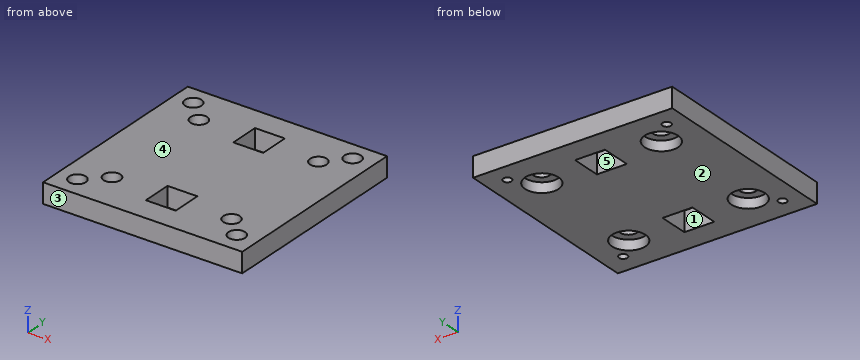
```python
from build123d import *

# Parameters (mm, degrees)
SKETCH044_W     = 100
SKETCH044_H     = 100
PAD009_DEPTH    = 10
SKETCH047_R     = 2.1
POCKET036_DEPTH = 10
SKETCH048_R     = 4.2
POCKET037_DEPTH = 5
SKETCH045_R     = 4.2
SKETCH045_W     = 15
SKETCH045_H     = 15
POCKET038_DEPTH = 10
SKETCH046_R     = 8.4
POCKET039_DEPTH = 5


with BuildPart() as part:
    # Sketch044 → Pad009 (new body)
    with BuildSketch(Plane.XY):
        with Locations((278.148773, 55.911007)):
            Rectangle(SKETCH044_W, SKETCH044_H)
    extrude(amount=PAD009_DEPTH)

    # Sketch047 → Pocket036 (cut)
    with BuildSketch(Plane.XY.offset(10)):
        with Locations((237.948565, 96.209783)):
            Circle(SKETCH047_R)
        with Locations((317.948565, 96.209783)):
            Circle(SKETCH047_R)
        with Locations((237.948565, 16.209783)):
            Circle(SKETCH047_R)
        with Locations((317.948565, 16.209783)):
            Circle(SKETCH047_R)
    extrude(amount=-POCKET036_DEPTH, mode=Mode.SUBTRACT)

    # Sketch048 (on Face5 of Pocket036) → Pocket037 (cut)
    with BuildSketch(Plane.XY.offset(10)):
        with Locations((237.975067, 96.170716)):
            Circle(SKETCH048_R)
        with Locations((317.975067, 96.170716)):
            Circle(SKETCH048_R)
        with Locations((237.975067, 16.170716)):
            Circle(SKETCH048_R)
        with Locations((317.975067, 16.170716)):
            Circle(SKETCH048_R)
    extrude(amount=-POCKET037_DEPTH, mode=Mode.SUBTRACT)

    # Sketch045 → Pocket038 (cut)
    with BuildSketch(Plane(origin=(-36, -54, 0), x_dir=(1, 0, 0), z_dir=(0, 0, 1))):
        with Locations((284.333469, 139.793406)):
            Circle(SKETCH045_R)
        with Locations((344.333469, 139.793406)):
            Circle(SKETCH045_R)
        with Locations((284.333469, 79.793406)):
            Circle(SKETCH045_R)
        with Locations((344.333469, 79.793406)):
            Circle(SKETCH045_R)
        with Locations((314.333469, 140.10933)):
            Rectangle(SKETCH045_W, SKETCH045_H)
        with Locations((314.333469, 79.675171)):
            Rectangle(SKETCH045_W, SKETCH045_H)
    extrude(amount=POCKET038_DEPTH, mode=Mode.SUBTRACT)

    # Sketch046 → Pocket039 (cut)
    with BuildSketch(Plane(origin=(-36, -54, 0), x_dir=(1, 0, 0), z_dir=(0, 0, 1))):
        with Locations((284.232884, 139.768659)):
            Circle(SKETCH046_R)
        with Locations((344.232884, 139.768659)):
            Circle(SKETCH046_R)
        with Locations((284.232884, 79.768659)):
            Circle(SKETCH046_R)
        with Locations((344.232884, 79.768659)):
            Circle(SKETCH046_R)
    extrude(amount=POCKET039_DEPTH, mode=Mode.SUBTRACT)


with BuildPart() as part_1:
    # Body005 placement: moved
    add(part.part.moved(Location((-277.9, -14.5, 317))))


solid = part_1.part
```
CAD build for the part. Positions are in the model's coordinates, mm. Face numbers are marked on the shaded views. A direction names the side the tool comes from. Coordinates: 2 decimals unless noted, no trailing zeros. Order: outer loops, then holes, each group sorted by start corner. A loop starts at its lowest first (then second) coordinate and runs counter-clockwise, first axis right, second up. Notation, with made-up numbers: (46, 23) -> (56, 23) arc R16 ccw to (56, 41) -> close; hole circle Ø7 at (37, -2). An arc over 180 degrees is marked (long way). Use one line per item in the form item = value. Start each with the question number.
1) Band-saw the part on A-A on x = 3.5. Give the cut face in (y, z).
2) Band-saw the part on C-C on z = 325.5. State how many separate pieces and enclosed holes the cut face has, then the cut area to 3 significant figures.
3) Drop flat-ended pins along their axis: pin 1 (5 mm diameter, centred on x = 28.5, y = 9, fed in from -Z); pin 2 (4 mm diameter, centred on x = -39.95, y = 1.71, fed in from +Z); pin 3 (5 mm diameter, centred on x = -39.92, y = 81.67, fed in from +Z). Give the stop position or say it passes through.
4) Drill centre lines: L1, parallel to Y at x = 3, z = 326; L2, parallel to X at y = 82, z = 324.5; L3, parallel to X at y = 6.5, z = 323.75. Where is each one in solid material? Low to high. Write a range as [from, to].
5) Pull direction Y, two halves, no side cores. Call the marked faces 1, 2 and 3: +Y half, -Y half, draft (parallel to the pull), parting line (faces both ways), or undercut.
6) Band-saw the part on D-D on x = -24. Give the cut face in (y, z).
7) Band-saw the part on B-B on y = 14. Give the cut face in (x, z).
8) Tool access for the marked faces 4 and 5: list every direction of +Z, -Z, +X, -X, +Y, -Y with a clear straight run to the whole face (end or side of a thin tool).
Entries:
q1.outline = (-8.59, 317) -> (3.68, 317) -> (3.68, 327) -> (-8.59, 327) -> close; (18.68, 317) -> (64.11, 317) -> (64.11, 327) -> (18.68, 327) -> close; (79.11, 317) -> (91.41, 317) -> (91.41, 327) -> (79.11, 327) -> close
q2.separate_pieces = 1
q2.enclosed_holes = 10
q2.area = 9,110 mm2
q3.pin_1 = 322
q3.pin_2 = through
q3.pin_3 = 322
q4.L1 = [-8.59, 3.68], [18.68, 64.11], [79.11, 91.41]
q4.L2 = [-49.75, -44.11], [-35.74, 35.89], [44.26, 50.25]
q4.L3 = [-49.75, -7.07], [7.93, 50.25]
q5.face_1 = undercut
q5.face_2 = draft
q5.face_3 = -Y half
q6.outline = (-8.59, 317) -> (5.07, 317) -> (5.07, 322) -> (17.47, 322) -> (17.47, 317) -> (65.07, 317) -> (65.07, 322) -> (77.47, 322) -> (77.47, 317) -> (91.41, 317) -> (91.41, 327) -> (-8.59, 327) -> close
q7.outline = (-49.75, 317) -> (-37.61, 317) -> (-37.61, 322) -> (-32.78, 322) -> (-32.78, 327) -> (-49.75, 327) -> close; (-26.35, 322) -> (-21.72, 322) -> (-21.72, 317) -> (-7.07, 317) -> (-7.07, 327) -> (-26.35, 327) -> close; (7.93, 317) -> (22.39, 317) -> (22.39, 322) -> (27.22, 322) -> (27.22, 327) -> (7.93, 327) -> close; (33.65, 322) -> (38.28, 322) -> (38.28, 317) -> (50.25, 317) -> (50.25, 327) -> (33.65, 327) -> close
q8.face_4 = +Z, +X, -X, +Y, -Y
q8.face_5 = +Z, -Z
